Input: part model. Units: mm. Frame: model coordinates. A direction names the side the tool comes from. Round coordinates to 2 decimals unless told otherwise and drop trailing zeros. Loops run counter-clockwise (first coordinate to the right, second up) from the corner with the lowest first, then second, coordinate; pieces in that order, holes last. Notation, with made-up numbers: (49.5, 32.5) - (70.5, 32.5) arc R23 ccw to (70.5, 63.5) - close; hole circle Ø7 at (13.5, 50.5). An arc over 180 degrees is marked (long way). Write each question's results on one line, items separated by ' | '.
from build123d import *

# Parameters (mm, degrees)
F0_W        = 39
F0_H        = 39
F0_R        = 0.975
F1_DEPTH    = 9
F2_T1_DEPTH = 62
F4_DEPTH    = 21
F5_DEPTH    = 21
F6_DEPTH    = 5.5
F7_DEPTH    = 1.5
F8_DEPTH    = 2.5
F9_DEPTH    = 1.5
F10_R       = 1.25
F11_DEPTH   = 2.5
F12_DEPTH   = 5
F13_DEPTH   = 1


# Not quite as in the source:
# - a fillet or chamfer that OpenCascade refuses, or shapes differently, is made with other operations: its cross-section is extruded or revolved along the edge and cut away or added


with BuildPart() as f1:
    # F0 (on Top) → F1 (new body)
    with BuildSketch(Plane.XY):
        Polygon((-2.625, 21), (-21, 21), (-21, -21), (-2.625, -21), (2.625, -21), (21, -21), (21, 21), (2.625, 21), align=None)
        Rectangle(F0_W, F0_H, mode=Mode.SUBTRACT)
        Rectangle(F0_W, F0_H)
        with BuildLine():
            ThreePointArc((16, 4.25), (16.6, 4.85), (17.2, 4.25))
            Line((17.2, 4.25), (17.2, -4.25))
            ThreePointArc((17.2, -4.25), (16.6, -4.85), (16, -4.25))
            Line((16, -4.25), (16, -6.5))
            ThreePointArc((16, -6.5), (16.6, -5.9), (17.2, -6.5))
            Line((17.2, -6.5), (17.2, -15.7))
            ThreePointArc((17.2, -15.7), (18.2606601718, -18.2606601718), (15.7, -17.2))
            Line((15.7, -17.2), (6.5, -17.2))
            ThreePointArc((6.5, -17.2), (5.9, -16.6), (6.5, -16))
            Line((6.5, -16), (4.25, -16))
            ThreePointArc((4.25, -16), (4.85, -16.6), (4.25, -17.2))
            Line((4.25, -17.2), (-4.25, -17.2))
            ThreePointArc((-4.25, -17.2), (-4.85, -16.6), (-4.25, -16))
            Line((-4.25, -16), (-6.5, -16))
            ThreePointArc((-6.5, -16), (-5.9, -16.6), (-6.5, -17.2))
            Line((-6.5, -17.2), (-15.7, -17.2))
            ThreePointArc((-15.7, -17.2), (-18.2606601718, -18.2606601718), (-17.2, -15.7))
            Line((-17.2, -15.7), (-17.2, -6.5))
            ThreePointArc((-17.2, -6.5), (-16.6, -5.9), (-16, -6.5))
            Line((-16, -6.5), (-16, -4.25))
            ThreePointArc((-16, -4.25), (-16.6, -4.85), (-17.2, -4.25))
            Line((-17.2, -4.25), (-17.2, 4.25))
            ThreePointArc((-17.2, 4.25), (-16.6, 4.85), (-16, 4.25))
            Line((-16, 4.25), (-16, 6.5))
            ThreePointArc((-16, 6.5), (-16.6, 5.9), (-17.2, 6.5))
            Line((-17.2, 6.5), (-17.2, 15.7))
            ThreePointArc((-17.2, 15.7), (-18.2606601718, 18.2606601718), (-15.7, 17.2))
            Line((-15.7, 17.2), (-6.5, 17.2))
            ThreePointArc((-6.5, 17.2), (-5.9, 16.6), (-6.5, 16))
            Line((-6.5, 16), (-4.25, 16))
            ThreePointArc((-4.25, 16), (-4.85, 16.6), (-4.25, 17.2))
            Line((-4.25, 17.2), (4.25, 17.2))
            ThreePointArc((4.25, 17.2), (4.85, 16.6), (4.25, 16))
            Line((4.25, 16), (6.5, 16))
            ThreePointArc((6.5, 16), (5.9, 16.6), (6.5, 17.2))
            Line((6.5, 17.2), (15.7, 17.2))
            ThreePointArc((15.7, 17.2), (18.2606601718, 18.2606601718), (17.2, 15.7))
            Line((17.2, 15.7), (17.2, 6.5))
            ThreePointArc((17.2, 6.5), (16.6, 5.9), (16, 6.5))
            Line((16, 6.5), (16, 4.25))
        make_face(mode=Mode.SUBTRACT)
        Polygon((16, -4.25), (16, 4.25), (16, 6.5), (16, 16), (6.5, 16), (4.25, 16), (-4.25, 16), (-6.5, 16), (-16, 16), (-16, 6.5), (-16, 4.25), (-16, -4.25), (-16, -6.5), (-16, -16), (-6.5, -16), (-4.25, -16), (4.25, -16), (6.5, -16), (16, -16), (16, -6.5), align=None)
        with Locations((-14, -14)):
            Circle(F0_R, mode=Mode.SUBTRACT)
        with Locations((14, -14)):
            Circle(F0_R, mode=Mode.SUBTRACT)
        with Locations((-14, 14)):
            Circle(F0_R, mode=Mode.SUBTRACT)
        Polygon((-8.75, 14), (0, 14), (0, 10.75), (-8.75, 10.75), (-9.75, 10.75), (-9.75, 14), align=None, mode=Mode.SUBTRACT)
        with BuildLine():
            Line((-8.75, 8.75), (8.75, 8.75))
            Line((8.75, 8.75), (8.75, 2.75))
            Line((8.75, 2.75), (10.75, 2.75))
            ThreePointArc((10.75, 2.75), (13.5, 0), (10.75, -2.75))
            Line((10.75, -2.75), (8.75, -2.75))
            Line((8.75, -2.75), (8.75, -8.75))
            Line((8.75, -8.75), (-8.75, -8.75))
            Line((-8.75, -8.75), (-8.75, -2.75))
            Line((-8.75, -2.75), (-10.75, -2.75))
            ThreePointArc((-10.75, -2.75), (-13.5, 0), (-10.75, 2.75))
            Line((-10.75, 2.75), (-8.75, 2.75))
            Line((-8.75, 2.75), (-8.75, 8.75))
        make_face(mode=Mode.SUBTRACT)
        Polygon((10.75, 3.8126846775), (10.75, 8.75), (10.75, 9.75), (14, 9.75), (14, 8.75), (14, 3.8126846775), align=None, mode=Mode.SUBTRACT)
        with Locations((14, 14)):
            Circle(F0_R, mode=Mode.SUBTRACT)
        Polygon((0, 10.75), (0, 14), (-8.75, 14), (-9.75, 14), (-9.75, 10.75), (-8.75, 10.75), align=None)
        Polygon((10.75, 9.75), (10.75, 8.75), (10.75, 3.8126846775), (14, 3.8126846775), (14, 8.75), (14, 9.75), align=None)
        with Locations((14, -14)):
            Circle(F0_R)
        with Locations((-14, -14)):
            Circle(F0_R)
        with Locations((-14, 14)):
            Circle(F0_R)
        with Locations((14, 14)):
            Circle(F0_R)
    extrude(amount=F1_DEPTH)

    # F2: fillet of radius 4 on 2 edges, made by hand

    # F2_s2 → F2_t1 (cut)
    with BuildSketch(Plane.XZ.offset(-31)):
        with BuildLine():
            ThreePointArc((-21, 5), (-19.8284271247, 7.8284271247), (-17, 9))
            Line((-17, 9), (-21, 9))
            Line((-21, 9), (-21, 5))
        make_face()
        with BuildLine():
            ThreePointArc((21, 5), (19.8284271247, 7.8284271247), (17, 9))
            Line((17, 9), (21, 9))
            Line((21, 9), (21, 5))
        make_face()
    extrude(amount=F2_T1_DEPTH, mode=Mode.SUBTRACT)

    # F3 (on Right) → F4 (join)
    with BuildSketch(Plane.YZ):
        Polygon((-21, 0), (-21, 1.25), (-23, 1.25), (-23, 4), (-24.5, 4), (-27.25, 1.25), (-27.25, -1.5), (-23, -1.5), (-21, -1.5), align=None)
    extrude(amount=F4_DEPTH)

    # F5 (add): a face of the model
    f5_faces = [f1.faces().sort_by_distance(p)[0] for p in [
        (0, -24.2579908676, 0.6723744292),
    ]]
    extrude(f5_faces, amount=F5_DEPTH)

    # F0 (on Top) → F6 (join)
    with BuildSketch(Plane.XY):
        with Locations((-14, -14)):
            Circle(F0_R)
        with Locations((14, -14)):
            Circle(F0_R)
        with Locations((-14, 14)):
            Circle(F0_R)
        with Locations((14, 14)):
            Circle(F0_R)
    extrude(amount=-F6_DEPTH)

    # F0 (on Top) → F7 (join)
    with BuildSketch(Plane.XY):
        Rectangle(F0_W, F0_H)
        with BuildLine():
            ThreePointArc((16, 4.25), (16.6, 4.85), (17.2, 4.25))
            Line((17.2, 4.25), (17.2, -4.25))
            ThreePointArc((17.2, -4.25), (16.6, -4.85), (16, -4.25))
            Line((16, -4.25), (16, -6.5))
            ThreePointArc((16, -6.5), (16.6, -5.9), (17.2, -6.5))
            Line((17.2, -6.5), (17.2, -15.7))
            ThreePointArc((17.2, -15.7), (18.2606601718, -18.2606601718), (15.7, -17.2))
            Line((15.7, -17.2), (6.5, -17.2))
            ThreePointArc((6.5, -17.2), (5.9, -16.6), (6.5, -16))
            Line((6.5, -16), (4.25, -16))
            ThreePointArc((4.25, -16), (4.85, -16.6), (4.25, -17.2))
            Line((4.25, -17.2), (-4.25, -17.2))
            ThreePointArc((-4.25, -17.2), (-4.85, -16.6), (-4.25, -16))
            Line((-4.25, -16), (-6.5, -16))
            ThreePointArc((-6.5, -16), (-5.9, -16.6), (-6.5, -17.2))
            Line((-6.5, -17.2), (-15.7, -17.2))
            ThreePointArc((-15.7, -17.2), (-18.2606601718, -18.2606601718), (-17.2, -15.7))
            Line((-17.2, -15.7), (-17.2, -6.5))
            ThreePointArc((-17.2, -6.5), (-16.6, -5.9), (-16, -6.5))
            Line((-16, -6.5), (-16, -4.25))
            ThreePointArc((-16, -4.25), (-16.6, -4.85), (-17.2, -4.25))
            Line((-17.2, -4.25), (-17.2, 4.25))
            ThreePointArc((-17.2, 4.25), (-16.6, 4.85), (-16, 4.25))
            Line((-16, 4.25), (-16, 6.5))
            ThreePointArc((-16, 6.5), (-16.6, 5.9), (-17.2, 6.5))
            Line((-17.2, 6.5), (-17.2, 15.7))
            ThreePointArc((-17.2, 15.7), (-18.2606601718, 18.2606601718), (-15.7, 17.2))
            Line((-15.7, 17.2), (-6.5, 17.2))
            ThreePointArc((-6.5, 17.2), (-5.9, 16.6), (-6.5, 16))
            Line((-6.5, 16), (-4.25, 16))
            ThreePointArc((-4.25, 16), (-4.85, 16.6), (-4.25, 17.2))
            Line((-4.25, 17.2), (4.25, 17.2))
            ThreePointArc((4.25, 17.2), (4.85, 16.6), (4.25, 16))
            Line((4.25, 16), (6.5, 16))
            ThreePointArc((6.5, 16), (5.9, 16.6), (6.5, 17.2))
            Line((6.5, 17.2), (15.7, 17.2))
            ThreePointArc((15.7, 17.2), (18.2606601718, 18.2606601718), (17.2, 15.7))
            Line((17.2, 15.7), (17.2, 6.5))
            ThreePointArc((17.2, 6.5), (16.6, 5.9), (16, 6.5))
            Line((16, 6.5), (16, 4.25))
        make_face(mode=Mode.SUBTRACT)
    extrude(amount=-F7_DEPTH)

    # F8 (cut): a face of the model
    f8_faces = [f1.faces().sort_by_distance(p)[0] for p in [
        (-18.9484567107, 0, -1.5),
    ]]
    extrude(f8_faces, amount=-F8_DEPTH, mode=Mode.SUBTRACT)

    # F0 (on Top) → F9 (join)
    with BuildSketch(Plane.XY):
        Polygon((-2.625, 21), (-21, 21), (-21, -21), (-2.625, -21), (2.625, -21), (21, -21), (21, 21), (2.625, 21), align=None)
        Rectangle(F0_W, F0_H, mode=Mode.SUBTRACT)
    extrude(amount=-F9_DEPTH)

    # F10 (on face) → F11 (cut)
    with BuildSketch(Plane(origin=(0, 0, -1.5), x_dir=(1, 0, 0), z_dir=(0, 0, -1))):
        with Locations((10.5, 24.75)):
            Circle(F10_R)
        with Locations((0, 24.75)):
            Circle(F10_R)
        with Locations((-10.5, 24.75)):
            Circle(F10_R)
    extrude(amount=-F11_DEPTH, mode=Mode.SUBTRACT)

    # F0 (on Top) → F12 (cut)
    with BuildSketch(Plane.XY):
        Polygon((10.75, 9.75), (10.75, 8.75), (10.75, 3.8126846775), (14, 3.8126846775), (14, 8.75), (14, 9.75), align=None)
        Polygon((0, 10.75), (0, 14), (-8.75, 14), (-9.75, 14), (-9.75, 10.75), (-8.75, 10.75), align=None)
    extrude(amount=F12_DEPTH, mode=Mode.SUBTRACT)

    # F0 (on Top) → F13 (cut)
    with BuildSketch(Plane.XY):
        Polygon((16, -4.25), (16, 4.25), (16, 6.5), (16, 16), (6.5, 16), (4.25, 16), (-4.25, 16), (-6.5, 16), (-16, 16), (-16, 6.5), (-16, 4.25), (-16, -4.25), (-16, -6.5), (-16, -16), (-6.5, -16), (-4.25, -16), (4.25, -16), (6.5, -16), (16, -16), (16, -6.5), align=None)
        with Locations((-14, -14)):
            Circle(F0_R, mode=Mode.SUBTRACT)
        with Locations((14, -14)):
            Circle(F0_R, mode=Mode.SUBTRACT)
        with Locations((-14, 14)):
            Circle(F0_R, mode=Mode.SUBTRACT)
        Polygon((-8.75, 14), (0, 14), (0, 10.75), (-8.75, 10.75), (-9.75, 10.75), (-9.75, 14), align=None, mode=Mode.SUBTRACT)
        with BuildLine():
            Line((-8.75, 8.75), (8.75, 8.75))
            Line((8.75, 8.75), (8.75, 2.75))
            Line((8.75, 2.75), (10.75, 2.75))
            ThreePointArc((10.75, 2.75), (13.5, 0), (10.75, -2.75))
            Line((10.75, -2.75), (8.75, -2.75))
            Line((8.75, -2.75), (8.75, -8.75))
            Line((8.75, -8.75), (-8.75, -8.75))
            Line((-8.75, -8.75), (-8.75, -2.75))
            Line((-8.75, -2.75), (-10.75, -2.75))
            ThreePointArc((-10.75, -2.75), (-13.5, 0), (-10.75, 2.75))
            Line((-10.75, 2.75), (-8.75, 2.75))
            Line((-8.75, 2.75), (-8.75, 8.75))
        make_face(mode=Mode.SUBTRACT)
        Polygon((10.75, 3.8126846775), (10.75, 8.75), (10.75, 9.75), (14, 9.75), (14, 8.75), (14, 3.8126846775), align=None, mode=Mode.SUBTRACT)
        with Locations((14, 14)):
            Circle(F0_R, mode=Mode.SUBTRACT)
    extrude(amount=F13_DEPTH, mode=Mode.SUBTRACT)


solid = f1.part
1. Line query: line 1 (Y direction, x = -10.5, z = 0.45); line 2 (X direction, y = -24.75, z = -1); line 3 (X direction, y = -11, z = 2.5). Output: solid intervals per line, ascending. Write a range as [from, to].
Answer:
line 1: [-27.25, -26], [-23.5, -19.5], [19.5, 21] | line 2: [-21, -11.75], [-9.25, -1.25], [1.25, 9.25], [11.75, 21] | line 3: [-21, -17.2], [-16, 16], [17.2, 21]
2. Section query A-A, the plane x = 8. Output: boundary loops of the cut face in (y, z).
Answer:
outline: (-27.25, -1.5) - (-19.5, -1.5) - (-19.5, 1) - (-17.2, 1) - (-17.2, 9) - (-21, 9) - (-21, 1.25) - (-23, 1.25) - (-23, 4) - (-24.5, 4) - (-27.25, 1.25) - close; (-16, 1) - (-8.75, 1) - (-8.75, 9) - (-16, 9) - close; (8.75, 1) - (16, 1) - (16, 9) - (8.75, 9) - close; (17.2, 1) - (19.5, 1) - (19.5, -1.5) - (21, -1.5) - (21, 9) - (17.2, 9) - close
3. Set-up query: faces 1 (the flat face through (0, 21, 4)), 2 (the cylindrical face through (5.9, -16.6, 5.1)), 3 (the cylindrical face through (9.25, -24.8, -0.27)). Return all of +Z, -Z, +X, -X, +Y, -Y with unobstructed straight access to the full face (end or side cutting, diameter ignored); none if empty.
Answer:
face 1: +Z, -Z, +X, -X, +Y | face 2: +Z, -Z | face 3: -Z
4. Section query B-B, the plane y = -18. Output: boundary loops of the cut face in (x, z).
Answer:
outline: (-21, -1.5) - (-19.5, -1.5) - (-19.5, 1) - (-18.47, 1) - (-18.47, 8.72) arc R4 ccw to (-21, 5) - close; (-15.93, 1) - (15.93, 1) - (15.93, 9) - (-15.93, 9) - close; (18.47, 1) - (19.5, 1) - (19.5, -1.5) - (21, -1.5) - (21, 5) arc R4 ccw to (18.47, 8.72) - close
5. Contact query for flat-ended pins moving along their axis: pin 1 (1 mm diameter, centred on x = 9.5, z = 3.5, fed in from -Y); pin 2 (5 mm diameter, centred on x = 8.5, y = 4.5, fed in from -Z); pin 3 (8 mm diameter, centred on x = -6.5, y = -18.5, fed in from -Z). Output: stop coordinate, or through.
Answer:
pin 1: y = -25.5 | pin 2: z = 1 | pin 3: z = -1.5
6. Section query C-C, the plane x = 12.5. Count the separate pieces of the cut face and the enclosed holes in it, plus the area to 3 significant figures.
Answer:
separate pieces: 4 | enclosed holes: 0 | area: 292 mm^2
7. Mould query, pull axis X, two halves, no side actions, for faces 4 (the flat face through (0, -27.25, 0)), 5 (the flat face through (0, 17.2, 5)), 6 (the flat face through (21, -3, 2)), 7 (the cylindrical face through (-11.75, -24.8, -0.27)). Classes: pulls with the +X half, pulls with the -X half, needs draft (parallel to the pull), parting line crosses it, or undercut.
Answer:
face 4: needs draft | face 5: undercut | face 6: pulls with the +X half | face 7: undercut
